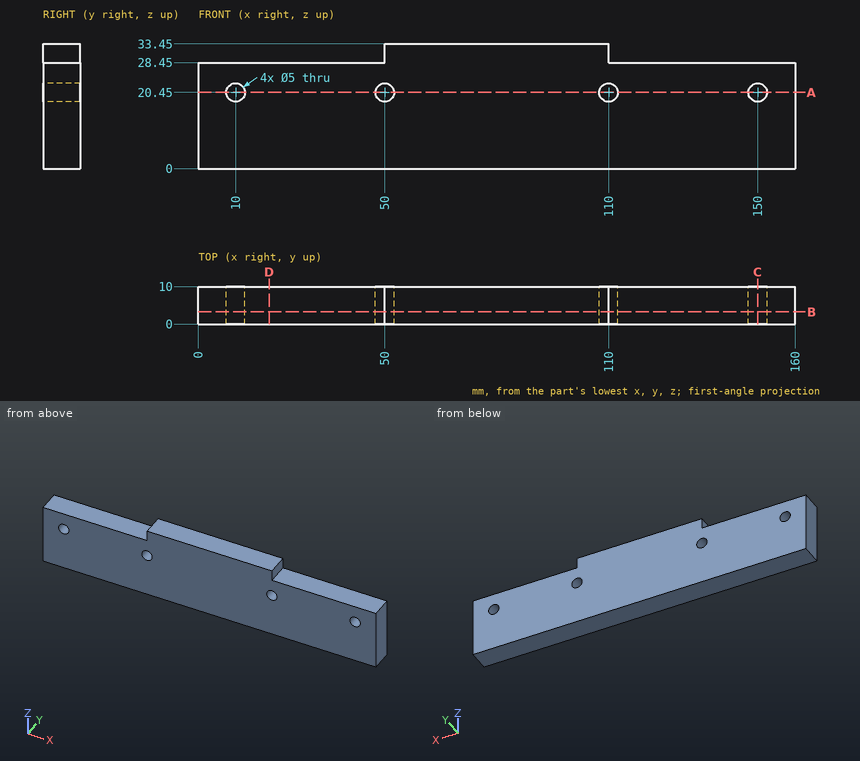
Drawing for the job (mm, zero at the part's lowest x, y, z). Coordinates: 2 decimals unless noted, no trailing zeros. Order: outer loops, then holes, each group sorted by start corner. A loop starts at its lowest first (then second) coordinate and runs counter-clockwise, first axis right, second up. Notation, with made-up numbers: (58.25, 10) -> (89.25, 10) arc R9 cw to (89.25, 26) -> close; hole circle Ø3 at (43, -31). An arc over 180 degrees is marked (long way). One line per item, written item: value.
(1) Slice it at A-A, the plane z = 20.45. List the corners of the cut face in (x, y), plus the area to 3 significant figures.
Checked values:
outline: (0, 0) -> (7.5, 0) -> (7.5, 10) -> (0, 10) -> close; (12.5, 0) -> (47.5, 0) -> (47.5, 10) -> (12.5, 10) -> close; (52.5, 0) -> (107.5, 0) -> (107.5, 10) -> (52.5, 10) -> close; (112.5, 0) -> (147.5, 0) -> (147.5, 10) -> (112.5, 10) -> close; (152.5, 0) -> (160, 0) -> (160, 10) -> (152.5, 10) -> close
area: 1,400 mm2
(2) Slice it at C-C, the plane x = 150. List the corners of the cut face in (y, z).
Checked values:
outline: (0, 0) -> (10, 0) -> (10, 17.95) -> (0, 17.95) -> close; (0, 22.95) -> (10, 22.95) -> (10, 28.45) -> (0, 28.45) -> close
(3) Drop flat-ended pins along their axis: pin 1 Ø3 at (x, z) = (50, 20.45) entering from -Y; pin 2 Ø1.5 at (y, z) = (2.5, 31) entering from -X; pin 3 Ø1.5 at (y, z) = (3.5, 30.5) entering from +X. Give the stop position or say it passes through.
Checked values:
pin 1: through
pin 2: x = 50
pin 3: x = 110
(4) Slice it at D-D, the plane x = 19. List the corners of the cut face in (y, z), plus the area to 4 significant figures.
Checked values:
outline: (0, 0) -> (10, 0) -> (10, 28.45) -> (0, 28.45) -> close
area: 284.5 mm2
(5) Probe line 1 (X direction, y = 7, z = 20.45); line 2 (Z direction, x = 150, y = 2); line 3 (X direction, y = 5, z = 29). List the from-to ranges inside material, lowest first. Write a range as [from, to].
Checked values:
line 1: [0, 7.5], [12.5, 47.5], [52.5, 107.5], [112.5, 147.5], [152.5, 160]
line 2: [0, 17.95], [22.95, 28.45]
line 3: [50, 110]
(6) Slice it at B-B, the plane y = 3.25. List the corners of the cut face in (x, z), plus the area to 3 significant figures.
Checked values:
outline: (0, 0) -> (160, 0) -> (160, 28.45) -> (110, 28.45) -> (110, 33.45) -> (50, 33.45) -> (50, 28.45) -> (0, 28.45) -> close; hole circle Ø5 at (10, 20.45); hole circle Ø5 at (50, 20.45); hole circle Ø5 at (110, 20.45); hole circle Ø5 at (150, 20.45)
area: 4,770 mm2
